Check sheet for the modelled part. Datum: model origin and axes. Units: mm. Face numbers are marked on the shaded views. Round coordinates to 2 decimals unless told otherwise and drop trailing zeros. Put each result on its own line as item: value. Start each with the question number.
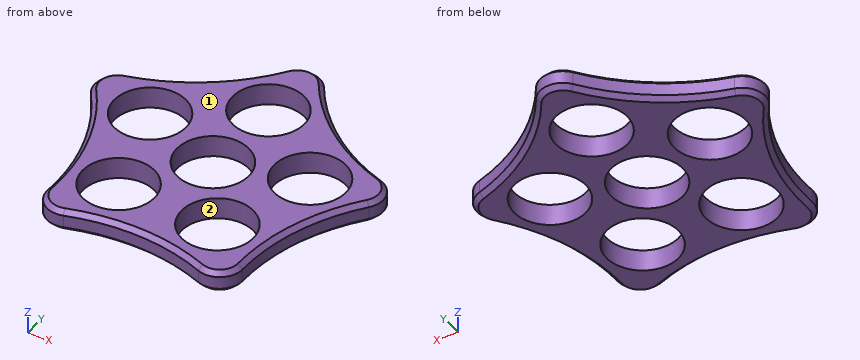
```python
from build123d import *

# Parameters (mm, degrees)
F0_R     = 8.001
F1_DEPTH = 4.826
F2_R     = 5.08
F3_SIZE  = 1.016


with BuildPart() as f1:
    # F0 (on Top) → F1 (new body)
    with BuildSketch(Plane.XY):
        with BuildLine():
            ThreePointArc((-37.4430950465, 12.1659990685), (-24.2528913362, -7.8802420857), (-23.1411053828, -31.8509990685))
            ThreePointArc((-23.1411053828, -31.8509990685), (0, -25.5009990685), (23.1411053828, -31.8509990685))
            ThreePointArc((23.1411053828, -31.8509990685), (24.2528913362, -7.8802420857), (37.4430950465, 12.1659990685))
            ThreePointArc((37.4430950465, 12.1659990685), (14.9891111712, 20.63074162), (0, 39.37))
            ThreePointArc((0, 39.37), (-14.9891111712, 20.63074162), (-37.4430950465, 12.1659990685))
        make_face()
        with Locations((-11.1973090562, -15.4117737428)):
            Circle(F0_R, mode=Mode.SUBTRACT)
        with Locations((11.1973090562, -15.4117737428)):
            Circle(F0_R, mode=Mode.SUBTRACT)
        Circle(F0_R, mode=Mode.SUBTRACT)
        with Locations((-18.1176266354, 5.8867737428)):
            Circle(F0_R, mode=Mode.SUBTRACT)
        with Locations((18.1176266354, 5.8867737428)):
            Circle(F0_R, mode=Mode.SUBTRACT)
        with Locations((0, 19.05)):
            Circle(F0_R, mode=Mode.SUBTRACT)
    extrude(amount=F1_DEPTH)

    # F2
    f2_edges = [f1.edges().sort_by_distance(p)[0] for p in [
        (0, 39.37, 2.413),
        (37.443095, 12.165999, 2.413),
        (23.141105, -31.850999, 2.413),
        (-23.141105, -31.850999, 2.413),
        (-37.443095, 12.165999, 2.413),
    ]]
    fillet(f2_edges, radius=F2_R)

    # F3
    f3_edges = [f1.edges().sort_by_distance(p)[0] for p in [
        (-32.297907, 10.494226, 0),
        (-24.252891, -7.880242, 4.826),
    ]]
    chamfer(f3_edges, length=F3_SIZE)


solid = f1.part
```
Q1. Depth check by flat-ended pin: pin 1 Ø2 at (y, z) = (-16.5, 3) entering from +X. Enter the tip coordinate at first touch or a pass-through.
Q2. Draft check along Y on the marked faces 1 and 2. Enter one of: +Y half, -Y half, draft (parallel to the pull), parting line (faces both ways), or undercut.
Q3. Material ranges on line 1 (X direction, y = -19, z = 3.7); line 2 (Y direction, x = 7, z = 0.35); line 3 (X direction, y = 10, z = 1.15), recorded low to high. Write a range as from..to.
Q4. Cross-section at A-A on x = 0. State how many separate pieces and enclosed holes the cut face has, and give its area (3 significant figures).
Answer list:
1. pin 1: stops at x = 22.49
2. face 1: draft
2. face 2: undercut
3. line 1: x = -22.13..-18.35, -4.05..4.05, 18.35..22.13
3. line 2: y = -25.37..-22.22, -8.6..-3.88, 3.88..15.17, 22.93..27.03
3. line 3: x = -32.43..-24.98, -11.25..11.25, 24.98..32.43
4. separate pieces: 3
4. enclosed holes: 0
4. area: 130 mm2
